from build123d import *

# Parameters (mm, degrees)
SKETCH1_W           = 80
SKETCH1_H           = 80
BOSS_EXTRUDE1_DEPTH = 1.5875
SKETCH2_OUTSIDE_W   = 104.636
SKETCH2_OUTSIDE_H   = 104.636
CUT_EXTRUDE2_DEPTH  = 10
SKETCH3_R           = 1.15
CUT_EXTRUDE3_DEPTH  = 57.657573413


with BuildPart() as part:
    # Sketch1 → Boss-Extrude1 (new, symmetric)
    with BuildSketch(Plane.XY):
        Rectangle(SKETCH1_W, SKETCH1_H)
    extrude(amount=BOSS_EXTRUDE1_DEPTH, both=True)

    # Sketch2 outside → Cut-Extrude2 (cut)
    with BuildSketch(Plane.XY.offset(1.5875)):
        Rectangle(SKETCH2_OUTSIDE_W, SKETCH2_OUTSIDE_H)
        Polygon((33.846153846, -36.825), (40, -36.825), (40, -31.159615385), (36.82, -31.159615385), (36.82, -25.494230769), (40, -25.494230769), (40, -19.828846154), (36.82, -19.828846154), (36.82, -14.163461538), (40, -14.163461538), (40, -8.498076923), (36.82, -8.498076923), (36.82, -2.832692308), (40, -2.832692308), (40, 2.832692308), (36.82, 2.832692308), (36.82, 8.498076923), (40, 8.498076923), (40, 14.163461538), (36.82, 14.163461538), (36.82, 19.828846154), (40, 19.828846154), (40, 25.494230769), (36.82, 25.494230769), (36.82, 31.159615385), (40, 31.159615385), (40, 36.825), (33.846153846, 36.825), (33.846153846, 40), (27.692307692, 40), (27.692307692, 36.825), (21.538461538, 36.825), (21.538461538, 40), (15.384615385, 40), (15.384615385, 36.825), (9.230769231, 36.825), (9.230769231, 40), (3.076923077, 40), (3.076923077, 36.825), (-3.076923077, 36.825), (-3.076923077, 40), (-9.230769231, 40), (-9.230769231, 36.825), (-15.384615385, 36.825), (-15.384615385, 40), (-21.538461538, 40), (-21.538461538, 36.825), (-27.692307692, 36.825), (-27.692307692, 40), (-33.846153846, 40), (-33.846153846, 36.825), (-40, 36.825), (-40, 31.159615385), (-36.82, 31.159615385), (-36.82, 25.494230769), (-40, 25.494230769), (-40, 19.828846154), (-36.82, 19.828846154), (-36.82, 14.163461538), (-40, 14.163461538), (-40, 8.498076923), (-36.82, 8.498076923), (-36.82, 2.832692308), (-40, 2.832692308), (-40, -2.832692308), (-36.82, -2.832692308), (-36.82, -8.498076923), (-40, -8.498076923), (-40, -14.163461538), (-36.82, -14.163461538), (-36.82, -19.828846154), (-40, -19.828846154), (-40, -25.494230769), (-36.82, -25.494230769), (-36.82, -31.159615385), (-40, -31.159615385), (-40, -36.825), (-33.846153846, -36.825), (-33.846153846, -40), (-27.692307692, -40), (-27.692307692, -36.825), (-21.538461538, -36.825), (-21.538461538, -40), (-15.384615385, -40), (-15.384615385, -36.825), (-9.230769231, -36.825), (-9.230769231, -40), (-3.076923077, -40), (-3.076923077, -36.825), (3.076923077, -36.825), (3.076923077, -40), (9.230769231, -40), (9.230769231, -36.825), (15.384615385, -36.825), (15.384615385, -40), (21.538461538, -40), (21.538461538, -36.825), (27.692307692, -36.825), (27.692307692, -40), (33.846153846, -40), align=None, mode=Mode.SUBTRACT)
    extrude(amount=-CUT_EXTRUDE2_DEPTH, mode=Mode.SUBTRACT)

    # Sketch3 → Cut-Extrude3 (cut, through all)
    with BuildSketch(Plane.XY.offset(1.5875)):
        Polygon((-13.65, -9.125), (-13.65, -28.125), (13.65, -28.125), (13.65, -9.125), (5, -9.125), (5, -4.825), (-5, -4.825), (-5, -9.125), align=None)
        with Locations((-10.284555817, -6.975)):
            Circle(SKETCH3_R)
        with Locations((10.284555817, -6.975)):
            Circle(SKETCH3_R)
        with Locations((-10.3, -29.875)):
            Circle(SKETCH3_R)
        with Locations((10.3, -29.875)):
            Circle(SKETCH3_R)
    extrude(amount=-CUT_EXTRUDE3_DEPTH, mode=Mode.SUBTRACT)


solid = part.part
Work out the finished part from the listing and answer in its coordinate system (mm). A direction names the side the tool comes from. Coordinates: 2 decimals unless noted, no trailing zeros. Write each loop counter-clockwise with the first axis right and the second up, starting at its lowest first coordinate (ties: lowest second). Pieces come first, ordered by that corner, then holes. Notation, with made-up numbers: M -17,7 L 22,7 A9 ccw 22,18 Z; hole C -17,-37.75 d6. An arc over 180 degrees is marked long. Answer as CSV lines item,"result". Start each with the question number.
Item 1: Section C-C on x = 10.3 is taken. Write down the section's boundary in (y, z) (1 decimal), and give its area (3 significant figures).
Item 2: Section D-D on x = -24.5 is taken. Write down the section's boundary in (y, z) (1 decimal), and give its area (3 significant figures).
Item 3: Section B-B on x = -4 is taken. Write down the section's boundary in (y, z) (1 decimal), and give its area (3 significant figures).
Item 4: A tool of negligible diameter and unlimited length cuts with its end or side. For faces 5 (the face through (-13.65, -18, 0)), 6 (the face through (-36.82, -6, 0)), 7 (the face through (3.077, -38, 0)), 8 (the face through (-33.846, 38, 0)), from which of +Z, -Z, +X, -X, +Y, -Y can it reach the whole face along a straight path? Write none if from no direction.
Item 5: Consider L1, parallel to X at y = -30, z = 0.95; L2, parallel to Y at x = 10.3, z = 0.3 (3 decimals); L3, parallel to X at y = -11, z = -0.3. Determine where each line is inside the solid, lowest interval first.
Item 6: Determine the mould class of faces 1 (the face through (-3.077, 38, 0)), 2 (the face through (-36.82, 28, 0)), 3 (the face through (25, -36.825, 0)), 4 (the face through (-5, -7, 0)) for opening direction Y: released by +Y, released by -Y, zero draft, split by the parting line, or undercut.
Item 7: Flat-ended cylindrical pins translate along their axes: P1, Ø1.6, axis at x = -1, z = -0.5, coming from the +Y side (3 decimals); P2, Ø1, axis at y = -29, z = -0.5, coming from the +X side; P3, Ø1, axis at x = -37, z = 0.5, coming from the -Y side (3 decimals). Find the tip coordinate at first contact, or state that the pin passes through.
Item 8: Section A-A on y = -16 is taken. Write down the section's boundary in (x, z), and give its area (3 significant figures).
Checks:
1,outline,"M -36.8,-1.6 L -31,-1.6 L -31,1.6 L -36.8,1.6 Z; M -28.7,-1.6 L -28.1,-1.6 L -28.1,1.6 L -28.7,1.6 Z; M -9.1,-1.6 L -8.1,-1.6 L -8.1,1.6 L -9.1,1.6 Z; M -5.8,-1.6 L 36.8,-1.6 L 36.8,1.6 L -5.8,1.6 Z"
1,area,"159 mm²"
2,outline,"M -36.8,-1.6 L 36.8,-1.6 L 36.8,1.6 L -36.8,1.6 Z"
2,area,"234 mm²"
3,outline,"M -40,-1.6 L -28.1,-1.6 L -28.1,1.6 L -40,1.6 Z; M -4.8,-1.6 L 40,-1.6 L 40,1.6 L -4.8,1.6 Z"
3,area,"180 mm²"
4,face 5,"+Z, -Z"
4,face 6,"+Z, -Z, -X"
4,face 7,"+Z, -Z, -Y"
4,face 8,"+Z, -Z, -X, +Y"
5,L1,"x = -36.82 to -11.44, -9.16 to 9.16, 11.44 to 36.82"
5,L2,"y = -36.825 to -31.025, -28.725 to -28.125, -9.125 to -8.125, -5.825 to 36.825"
5,L3,"x = -40 to -13.65, 13.65 to 40"
6,face 1,"zero draft"
6,face 2,"undercut"
6,face 3,"released by -Y"
6,face 4,"undercut"
7,P1,"stops at y = 36.825"
7,P2,"stops at x = 36.82"
7,P3,"stops at y = -36.825"
8,outline,"M -36.82,-1.59 L -13.65,-1.59 L -13.65,1.59 L -36.82,1.59 Z; M 13.65,-1.59 L 36.82,-1.59 L 36.82,1.59 L 13.65,1.59 Z"
8,area,"147 mm²"
